Verification items for the finished model (mm, model axes). Face numbers are marked on the shaded views. A direction names the side the tool comes from. Round coordinates to 2 decimals unless told otherwise and drop trailing zeros. Write each loop counter-clockwise with the first axis right and the second up, starting at its lowest first coordinate (ties: lowest second). Pieces come first, ordered by that corner, then holes. Notation, with made-up numbers: (7, -20.5) - (56, -20.5) arc R6 ccw to (56, -11.5) - close; hole circle Ø7 at (-14, 0). An arc over 180 degrees is marked (long way). Answer as a JSON object with one key per item and string values. Group by question number.
1) Section check C-C (z = 18.25). Enter the section's corners in (x, y), then the cut area to 3 significant figures.
2) Section check D-D (y = 32). Enter the section's corners in (x, z), then the cut area to 3 significant figures.
3) Section check B-B (y = 51.5). Enter the section's corners in (x, z), then the cut area to 3 significant figures.
4) Section check A-A (y = 38.5). Enter the section's corners in (x, z).
5) Go/stop test with flat-tipped pins: pin 1 Ø2 at (x, z) = (12, 3) entering from -Y; pin 2 Ø2 at (x, y) = (0, 20) entering from -Z; pin 3 Ø8 at (y, z) = (44, 13.5) entering from -X; pin 4 Ø10 at (x, y) = (-7, 31) entering from -Z. Record where each tip stops, or that it passes through.
6) Set-up check for the marked faces 1 and 2: record each of +Z, -Z, +X, -X, +Y, -Y from which the full face is reachable in a straight line by a thin tool's end or side.
7) Thickness scan on line 1 (X direction, y = 32, z = 4.3); line 2 (Y direction, x = -1, z = 5.5); line 3 (Z direction, x = -12, y = 6). Record the ranges inside material, lowest first.
8) Mould release check, pull along X, two halves, no side actions. Record for the marked faces 3, 4, 5 and 6: +X half, -X half, draft (parallel to the pull), parting line (faces both ways), or undercut.
```python
from build123d import *

# Parameters (mm, degrees)
ESBO_O1_W                                            = 38
ESBO_O1_H                                            = 56
ESBO_O1_R                                            = 4
RESSALTO_EXTRUS_O1_DEPTH                             = 6
ESBO_O6_R                                            = 16.54
CORTE_EXTRUS_O5_DEPTH                                = 4
ESBO_O7_R                                            = 4
ESBO_O7_R_2                                          = 1.25
CORTE_EXTRUS_O6_DEPTH                                = 60.270566051
ESCAREADO_PARA_PARAFUSO_DE_M_QUINA_COM_C_D           = 2.9
ESCAREADO_PARA_PARAFUSO_DE_M_QUINA_COM_C_CSINK_D     = 5.5
ESCAREADO_PARA_PARAFUSO_DE_M_QUINA_COM_C_CSINK_ANGLE = 90
RESSALTO_EXTRUS_O2_DEPTH                             = 4
RESSALTO_EXTRUS_O3_DEPTH                             = 5.79
ESBO_O17_R                                           = 3.5
RESSALTO_EXTRUS_O4_DEPTH                             = 7
ESBO_O18_R                                           = 2
RESSALTO_EXTRUS_O5_DEPTH                             = 4
CHANFRO1_SIZE                                        = 4
CHANFRO1_SIZE_2                                      = 5.29
FURO_ROSCADO_DE_M3X0_51_D                            = 2.5
FURO_ROSCADO_DE_M3X0_51_DEPTH                        = 10
FURO_ROSCADO_DE_M3X0_51_TIP                          = 0.751075774
FURO_ROSCADO_DE_M3X0_52_D                            = 2.5
FURO_ROSCADO_DE_M3X0_52_DEPTH                        = 8.5
FURO_ROSCADO_DE_M3X0_52_TIP                          = 0.751075774
FURO_ROSCADO_DE_M3X0_53_D                            = 2.5
FURO_ROSCADO_DE_M3X0_53_DEPTH                        = 6
FURO_ROSCADO_DE_M3X0_53_TIP                          = 0.751075774
CHANFRO2_SIZE                                        = 1


with BuildPart() as part:
    # Esboço1 → Ressalto-extrusão1 (new body)
    with BuildSketch(Plane.XY):
        with Locations((0, 28)):
            Rectangle(ESBO_O1_W, ESBO_O1_H)
        with Locations((0, 20)):
            Circle(ESBO_O1_R, mode=Mode.SUBTRACT)
    extrude(amount=RESSALTO_EXTRUS_O1_DEPTH)

    # Esboço6 → Corte-extrusão5 (cut)
    with BuildSketch(Plane(origin=(0, 0, 0), x_dir=(-1, 0, 0), z_dir=(0, 0, -1))):
        with Locations((0, 38.5)):
            Circle(ESBO_O6_R)
    extrude(amount=-CORTE_EXTRUS_O5_DEPTH, mode=Mode.SUBTRACT)

    # Esboço7 → Corte-extrusão6 (cut, through all)
    with BuildSketch(Plane(origin=(0, 0, 4), x_dir=(-1, 0, 0), z_dir=(0, 0, -1))):
        with Locations((0, 38.5)):
            Circle(ESBO_O7_R)
        with Locations((11.258330249, 32)):
            Circle(ESBO_O7_R_2)
        with Locations((-11.258330249, 32)):
            Circle(ESBO_O7_R_2)
        with Locations((0, 51.5)):
            Circle(ESBO_O7_R_2)
    extrude(amount=-CORTE_EXTRUS_O6_DEPTH, mode=Mode.SUBTRACT)

    # Escareado para parafuso de máquina com cabeça chata de M2.51 (through all)
    with Locations(Plane.XY.offset(6)):
        with Locations((0, 51.5), (11.258330249, 32), (-11.258330249, 32)):
            CounterSinkHole(ESCAREADO_PARA_PARAFUSO_DE_M_QUINA_COM_C_D / 2, ESCAREADO_PARA_PARAFUSO_DE_M_QUINA_COM_C_CSINK_D / 2, counter_sink_angle=ESCAREADO_PARA_PARAFUSO_DE_M_QUINA_COM_C_CSINK_ANGLE)

    # Esboço15 → Ressalto-extrusão2 (add)
    with BuildSketch(Plane(origin=(0, 0, 0), x_dir=(-1, 0, 0), z_dir=(0, 0, -1))):
        with BuildLine():
            ThreePointArc((-3.280592218, 22.288605405), (0, 16), (3.280592218, 22.288605405))
            ThreePointArc((3.280592218, 22.288605405), (0, 21.96), (-3.280592218, 22.288605405))
        make_face()
    extrude(amount=-RESSALTO_EXTRUS_O2_DEPTH)

    # Esboço16 → Ressalto-extrusão3 (add)
    with BuildSketch(Plane.XY.offset(4)):
        with BuildLine():
            ThreePointArc((-3.280592218, 22.288605405), (0, 16), (3.280592218, 22.288605405))
            ThreePointArc((3.280592218, 22.288605405), (0, 24), (-3.280592218, 22.288605405))
        make_face()
    extrude(amount=RESSALTO_EXTRUS_O3_DEPTH)

    # Esboço17 → Ressalto-extrusão4 (add)
    with BuildSketch(Plane.XY.offset(9.79)):
        with Locations((0, 20)):
            Circle(ESBO_O17_R)
    extrude(amount=RESSALTO_EXTRUS_O4_DEPTH)

    # Esboço18 → Ressalto-extrusão5 (add)
    with BuildSketch(Plane.XY.offset(16.79)):
        with Locations((0, 20)):
            Circle(ESBO_O18_R)
    extrude(amount=RESSALTO_EXTRUS_O5_DEPTH)

    # Chanfro1
    # the kernel refuses this chamfer: 5.29, 4 mm, written as the material it adds along each edge
    with BuildSketch(Plane(origin=(0, 20, 6), x_dir=(0.8201480544065356, 0.5721513513513485, 0), z_dir=(-0.5721513513513485, 0.8201480544065356, 0))) as chanfro1_piece_1_section:
        Polygon((4 + CHANFRO1_SIZE, 0), (4, -CHANFRO1_SIZE_2), (4, 0), align=None)
    chanfro1_piece_1 = revolve(axis=Axis((0, 20, 6), (0, 0, -1)), mode=Mode.PRIVATE)
    chanfro1_piece_1 = split(chanfro1_piece_1, bisect_by=Plane(origin=(-5.391672126, 16.23866389, 9.79), z_dir=(0, 0, -1)), keep=Keep.TOP, mode=Mode.PRIVATE)
    add(chanfro1_piece_1)

    # Furo roscado de M3x0.51
    with Locations(Plane.XY.offset(20.79)):
        with Locations((0, 20)):
            Hole(FURO_ROSCADO_DE_M3X0_51_D / 2, depth=FURO_ROSCADO_DE_M3X0_51_DEPTH)
            with Locations((0, 0, -(FURO_ROSCADO_DE_M3X0_51_DEPTH + FURO_ROSCADO_DE_M3X0_51_TIP / 2))):  # 118° drill point
                Cone(0, FURO_ROSCADO_DE_M3X0_51_D / 2, FURO_ROSCADO_DE_M3X0_51_TIP, mode=Mode.SUBTRACT)

    # Furo roscado de M3x0.52
    with Locations(Plane(origin=(0, 0, 0), x_dir=(-1, 0, 0), z_dir=(0, -1, 0))):
        with Locations((12, -3), (0, -3), (-12, -3)):
            Hole(FURO_ROSCADO_DE_M3X0_52_D / 2, depth=FURO_ROSCADO_DE_M3X0_52_DEPTH)
            with Locations((0, 0, -(FURO_ROSCADO_DE_M3X0_52_DEPTH + FURO_ROSCADO_DE_M3X0_52_TIP / 2))):  # 118° drill point
                Cone(0, FURO_ROSCADO_DE_M3X0_52_D / 2, FURO_ROSCADO_DE_M3X0_52_TIP, mode=Mode.SUBTRACT)

    # Furo roscado de M3x0.53
    with Locations(Plane(origin=(0, 56, 0), x_dir=(1, 0, 0), z_dir=(0, 1, 0))):
        with Locations((-14, -3), (14, -3)):
            Hole(FURO_ROSCADO_DE_M3X0_53_D / 2, depth=FURO_ROSCADO_DE_M3X0_53_DEPTH)
            with Locations((0, 0, -(FURO_ROSCADO_DE_M3X0_53_DEPTH + FURO_ROSCADO_DE_M3X0_53_TIP / 2))):  # 118° drill point
                Cone(0, FURO_ROSCADO_DE_M3X0_53_D / 2, FURO_ROSCADO_DE_M3X0_53_TIP, mode=Mode.SUBTRACT)

    # Chanfro2
    chanfro2_edges = [part.edges().sort_by_distance(p)[0] for p in [
        (4, 38.5, 6),
    ]]
    chamfer(chanfro2_edges, length=CHANFRO2_SIZE)


solid = part.part
```
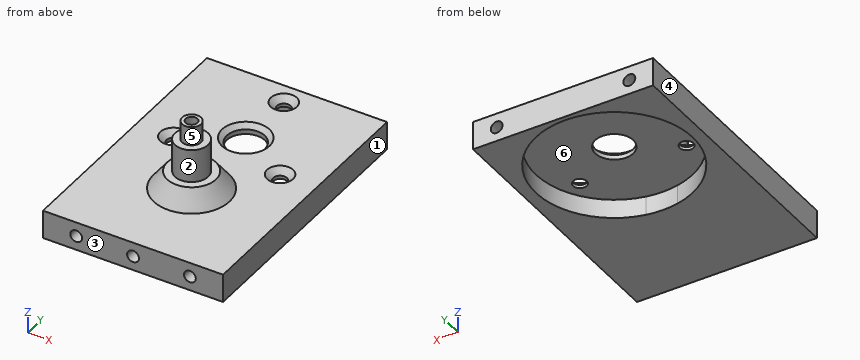
Returned:
{
 "1": {"outline": "circle Ø4 at (0, 20); hole circle Ø2.5 at (0, 20)", "area": "7.66 mm2"},
 "2": {"outline": "(-19, 0) - (-15.21, 0) - (-15.21, 4) - (-12.71, 4) - (-12.71, 4.7) - (-14.01, 6) - (-19, 6) - close; (-9.81, 4) - (9.81, 4) - (9.81, 4.7) - (8.51, 6) - (-8.51, 6) - (-9.81, 4.7) - close; (12.71, 4) - (15.21, 4) - (15.21, 0) - (19, 0) - (19, 6) - (14.01, 6) - (12.71, 4.7) - close", "area": "91.3 mm2"},
 "3": {"outline": "(-19, 0) - (-10.23, 0) - (-10.23, 4) - (-1.45, 4) - (-1.45, 4.7) - (-2.75, 6) - (-19, 6) - close; (1.45, 4) - (10.23, 4) - (10.23, 0) - (19, 0) - (19, 6) - (2.75, 6) - (1.45, 4.7) - close; hole circle Ø2.5 at (-14, 3); hole circle Ø2.5 at (14, 3)", "area": "129 mm2"},
 "4": {"outline": "(-19, 0) - (-16.54, 0) - (-16.54, 4) - (-4, 4) - (-4, 5) - (-5, 6) - (-19, 6) - close; (4, 4) - (16.54, 4) - (16.54, 0) - (19, 0) - (19, 6) - (5, 6) - (4, 5) - close"},
 "5": {"pin 1": "y = 8.65", "pin 2": "z = 0", "pin 3": "through", "pin 4": "z = 4"},
 "6": {"face 1": "+Z, -Z, +X, +Y, -Y", "face 2": "+Z"},
 "7": {"line 1": "-19 to -12.71, -9.81 to 9.81, 12.71 to 19", "line 2": "0 to 34.11, 42.89 to 49.48, 53.52 to 56", "line 3": "0 to 1.75, 4.25 to 6"},
 "8": {"face 3": "draft", "face 4": "-X half", "face 5": "parting line", "face 6": "undercut"}
}
